Design review of the part built by this model. Coordinates are the model's own, in mm. A direction names the side the tool comes from. Coordinates: 2 decimals unless noted, no trailing zeros. Loops run counter-clockwise (first coordinate to the right, second up) from the corner with the lowest first, then second, coordinate; pieces in that order, holes last. Notation, with made-up numbers: (-13, 36) - (26, 36) arc R13 ccw to (26, 54) - close; hole circle Ø10 at (38, -5.5). An arc over 180 degrees is marked (long way). Use one line per item in the form item = value. Start each with the question number.
(1) Add section B-B (x = 131). State the section outline as (y, z) points, plus the area to 3 significant figures.
(2) The part is to be moulded in two halves that separate along Z. For faces 1 (the face through (0, 1, -74)), 2 (the face through (41.95, -3.72, -14.14)), 3 (the face through (41.95, -3.72, -54.24)), 4 (the face through (33, -4, -144.797)), say which applies: pulls with the +Z half, pulls with the -Z half, needs draft (parallel to the pull), parting line crosses it, or undercut.
(3) Add section A-A (y = -5.25). Count the separate pieces of the cut face and the enclosed holes in it, plus the area to 3 significant figures.
(4) Tool access review of faces 5 (the face through (67, -4, -95)), 6 (the face through (33, -4, -110.397)), 7 (the face through (115, -4, -3.33)), 8 (the face through (95.5, -3.7, -17.4)): name each direction out of +Z, -Z, +X, -X, +Y, -Y from which nothing blocks a thin tool from reaching the whole face with its end or side.
(5) For L1, parallel to Z at x = 50, y = -4; L2, parallel to Z at x = 89, y = -5; L3, parallel to X at y = -6, z = -56.5, list the stretches that pass through material, from the lowest coordinate up.
(6) Add section C-C (z = -102). State the section outline as (x, y) points, plus the area to 3 significant figures.
(7) Clearance check with flat-ended pins moving along their axes: pin 1 Ø2.5 at (x, y) = (117.5, -2) entering from +Z; pin 2 Ø1.1 at (x, z) = (32, -14.5) entering from -Y; pin 3 Ø1.5 at (y, z) = (-4, -83.5) entering from +X. State where each tip first meets the part, or that it passes through.
```python
from build123d import *

# Parameters (mm, degrees)
SKETCH2_W           = 149
SKETCH2_H           = 148.13
BOSS_EXTRUDE1_DEPTH = 4
SKETCH3_W           = 67
SKETCH3_H           = 24.5
SKETCH3_H_2         = 30.2
SKETCH3_H_3         = 30.1967
BOSS_EXTRUDE3_DEPTH = 11.55
FILLET1_R           = 2


with BuildPart() as part:
    # Sketch2 → Boss-Extrude1 (new body)
    with BuildSketch(Plane(origin=(0, 0, 0), x_dir=(1, 0, 0), z_dir=(0, 1, 0))):
        with Locations((74.5, 74.065)):
            Rectangle(SKETCH2_W, SKETCH2_H)
    extrude(amount=BOSS_EXTRUDE1_DEPTH)

    # Sketch3 → Boss-Extrude3 (add)
    # profile 1 of 8: a face of its own
    with BuildSketch(Plane(origin=(0, 4, 0), x_dir=(1, 0, 0), z_dir=(0, 1, 0))):
        with Locations((33.5, 132.5467)):
            Rectangle(SKETCH3_W, SKETCH3_H)
        with BuildLine():
            ThreePointArc((12.85, 133.7967), (11.025, 135.6217), (12.85, 137.4467))
            Line((12.85, 137.4467), (40.15, 137.4467))
            ThreePointArc((40.15, 137.4467), (41.975, 135.6217), (40.15, 133.7967))
            Line((40.15, 133.7967), (12.85, 133.7967))
        make_face(mode=Mode.SUBTRACT)
    # profile 2 of 8: a face of its own
    with BuildSketch(Plane(origin=(0, 4, 0), x_dir=(1, 0, 0), z_dir=(0, 1, 0))):
        with Locations((115.5, 135.88)):
            Rectangle(SKETCH3_W, SKETCH3_H)
        with BuildLine():
            ThreePointArc((97.3, 136.48), (95.475, 138.305), (97.3, 140.13))
            Line((97.3, 140.13), (124.6, 140.13))
            ThreePointArc((124.6, 140.13), (126.425, 138.305), (124.6, 136.48))
            Line((124.6, 136.48), (97.3, 136.48))
        make_face(mode=Mode.SUBTRACT)
    # profile 3 of 8: a face of its own
    with BuildSketch(Plane(origin=(0, 4, 0), x_dir=(1, 0, 0), z_dir=(0, 1, 0))):
        with Locations((33.5, 95.2967)):
            Rectangle(SKETCH3_W, SKETCH3_H_2)
        with BuildLine():
            ThreePointArc((12.85, 92.4967), (11.05, 94.2967), (12.85, 96.0967))
            Line((12.85, 96.0967), (40.15, 96.0967))
            ThreePointArc((40.15, 96.0967), (41.95, 94.2967), (40.15, 92.4967))
            Line((40.15, 92.4967), (12.85, 92.4967))
        make_face(mode=Mode.SUBTRACT)
    # profile 4 of 8: a face of its own
    with BuildSketch(Plane(origin=(0, 4, 0), x_dir=(1, 0, 0), z_dir=(0, 1, 0))):
        with Locations((115.5, 98.63)):
            Rectangle(SKETCH3_W, SKETCH3_H_2)
        with BuildLine():
            ThreePointArc((97.3, 95.83), (95.5, 97.63), (97.3, 99.43))
            Line((97.3, 99.43), (124.6, 99.43))
            ThreePointArc((124.6, 99.43), (126.4, 97.63), (124.6, 95.83))
            Line((124.6, 95.83), (97.3, 95.83))
        make_face(mode=Mode.SUBTRACT)
    # profile 5 of 8: a face of its own
    with BuildSketch(Plane(origin=(0, 4, 0), x_dir=(1, 0, 0), z_dir=(0, 1, 0))):
        with Locations((33.5, 55.1967)):
            Rectangle(SKETCH3_W, SKETCH3_H_2)
        with BuildLine():
            ThreePointArc((12.85, 52.3967), (11.05, 54.1967), (12.85, 55.9967))
            Line((12.85, 55.9967), (40.15, 55.9967))
            ThreePointArc((40.15, 55.9967), (41.95, 54.1967), (40.15, 52.3967))
            Line((40.15, 52.3967), (12.85, 52.3967))
        make_face(mode=Mode.SUBTRACT)
    # profile 6 of 8: a face of its own
    with BuildSketch(Plane(origin=(0, 4, 0), x_dir=(1, 0, 0), z_dir=(0, 1, 0))):
        with Locations((115.5, 58.53)):
            Rectangle(SKETCH3_W, SKETCH3_H_2)
        with BuildLine():
            ThreePointArc((97.3, 55.73), (95.5, 57.53), (97.3, 59.33))
            Line((97.3, 59.33), (124.6, 59.33))
            ThreePointArc((124.6, 59.33), (126.4, 57.53), (124.6, 55.73))
            Line((124.6, 55.73), (97.3, 55.73))
        make_face(mode=Mode.SUBTRACT)
    # profile 7 of 8: a face of its own
    with BuildSketch(Plane(origin=(0, 4, 0), x_dir=(1, 0, 0), z_dir=(0, 1, 0))):
        with Locations((33.5, 15.09835)):
            Rectangle(SKETCH3_W, SKETCH3_H_3)
        with BuildLine():
            ThreePointArc((12.85, 12.2967), (11.05, 14.0967), (12.85, 15.8967))
            Line((12.85, 15.8967), (40.15, 15.8967))
            ThreePointArc((40.15, 15.8967), (41.95, 14.0967), (40.15, 12.2967))
            Line((40.15, 12.2967), (12.85, 12.2967))
        make_face(mode=Mode.SUBTRACT)
    # profile 8 of 8: a face of its own
    with BuildSketch(Plane(origin=(0, 4, 0), x_dir=(1, 0, 0), z_dir=(0, 1, 0))):
        with Locations((115.5, 18.43)):
            Rectangle(SKETCH3_W, SKETCH3_H_2)
        with BuildLine():
            ThreePointArc((97.3, 15.63), (95.5, 17.43), (97.3, 19.23))
            Line((97.3, 19.23), (124.6, 19.23))
            ThreePointArc((124.6, 19.23), (126.4, 17.43), (124.6, 15.63))
            Line((124.6, 15.63), (97.3, 15.63))
        make_face(mode=Mode.SUBTRACT)
    extrude(amount=-BOSS_EXTRUDE3_DEPTH)

    # Fillet1
    fillet1_edges = [part.edges().sort_by_distance(p)[0] for p in [
        (67, -3.775, -110.3967),
        (67, -3.775, -80.1967),
        (0, -3.775, -80.1967),
        (0, -3.775, -110.3967),
        (82, -3.775, -113.73),
        (149, -3.775, -113.73),
        (149, -3.775, -83.53),
        (82, -3.775, -83.53),
        (67, -3.775, -70.2967),
        (67, -3.775, -40.0967),
        (0, -3.775, -40.0967),
        (0, -3.775, -70.2967),
        (82, -3.775, -73.63),
        (149, -3.775, -73.63),
        (149, -3.775, -43.43),
        (82, -3.775, -43.43),
        (67, -3.775, -30.1967),
        (67, -3.775, 0),
        (0, -3.775, -30.1967),
        (67, -3.775, -144.7967),
        (67, -3.775, -120.2967),
        (0, -3.775, -120.2967),
        (0, -3.775, -144.7967),
        (82, -3.775, -33.53),
        (149, -3.775, -33.53),
        (149, -3.775, -3.33),
        (82, -3.775, -3.33),
        (82, -3.775, -148.13),
        (149, -3.775, -123.63),
        (82, -3.775, -123.63),
        (149, -1.775, -148.13),
        (0, -1.775, 0),
    ]]
    fillet(fillet1_edges, radius=FILLET1_R)


solid = part.part
```
Computed values:
q1.outline = (-7.55, -148.13) - (4, -148.13) - (4, 0) - (0, 0) - (0, -3.33) - (-7.55, -3.33) - (-7.55, -33.53) - (0, -33.53) - (0, -43.43) - (-7.55, -43.43) - (-7.55, -73.63) - (0, -73.63) - (0, -83.53) - (-7.55, -83.53) - (-7.55, -113.73) - (0, -113.73) - (0, -123.63) - (-7.55, -123.63) - close
q1.area = 1,460 mm^2
q2.face_1 = needs draft
q2.face_2 = undercut
q2.face_3 = undercut
q2.face_4 = pulls with the -Z half
q3.separate_pieces = 8
q3.enclosed_holes = 8
q3.area = 14,500 mm^2
q4.face_5 = +Z, -Z, -Y
q4.face_6 = -X, -Y
q4.face_7 = +Z, +X, -Y
q4.face_8 = -Y
q5.L1 = -144.8 to -120.3, -110.4 to -80.2, -70.3 to -40.1, -30.2 to 0
q5.L2 = -148.13 to -123.63, -113.73 to -83.53, -73.63 to -43.43, -33.53 to -3.33
q5.L3 = 0 to 67, 82 to 95.82, 126.08 to 149
q6.outline = (0, -7.55) - (67, -7.55) - (67, 0) - (82, 0) - (82, -7.55) - (149, -7.55) - (149, 4) - (0, 4) - close
q6.area = 1,610 mm^2
q7.pin_1 = -3.33
q7.pin_2 = 0
q7.pin_3 = 148.54
